```python
from build123d import *

# Parameters (mm, degrees)
SKETCH1_W           = 6.35
SKETCH1_H           = 241.3
BOSS_EXTRUDE1_DEPTH = 71.12
SKETCH2_W           = 6.35
SKETCH2_H           = 22.86
SKETCH2_H_2         = 25.4
CUT_EXTRUDE1_DEPTH  = 6.35
SKETCH3_W           = 6.35
SKETCH3_H           = 50.8
SKETCH3_H_2         = 25.4
CUT_EXTRUDE2_DEPTH  = 6.35
SKETCH4_W           = 19.05
SKETCH4_H           = 19.05
CUT_EXTRUDE3_DEPTH  = 7.35


with BuildPart() as part:
    # Sketch1 → Boss-Extrude1 (new body)
    with BuildSketch(Plane.XY):
        with Locations((-136.525, -120.65)):
            Rectangle(SKETCH1_W, SKETCH1_H)
    extrude(amount=-BOSS_EXTRUDE1_DEPTH)

    # Sketch2 → Cut-Extrude1 (cut)
    with BuildSketch(Plane(origin=(-133.35, 0, 0), x_dir=(0, 0, -1), z_dir=(1, 0, 0))):
        with Locations((67.945, -38.1)):
            Rectangle(SKETCH2_W, SKETCH2_H)
        with Locations((67.945, -87.63)):
            Rectangle(SKETCH2_W, SKETCH2_H_2)
        with Locations((67.945, -138.43)):
            Rectangle(SKETCH2_W, SKETCH2_H_2)
        with Locations((67.945, -201.93)):
            Rectangle(SKETCH2_W, SKETCH2_H_2)
    extrude(amount=-CUT_EXTRUDE1_DEPTH, mode=Mode.SUBTRACT)

    # Sketch3 → Cut-Extrude2 (cut)
    with BuildSketch(Plane(origin=(-133.35, 0, 0), x_dir=(0, 0, -1), z_dir=(1, 0, 0))):
        with Locations((3.175, -190.5)):
            Rectangle(SKETCH3_W, SKETCH3_H)
        with Locations((3.175, -127)):
            Rectangle(SKETCH3_W, SKETCH3_H_2)
        with Locations((3.175, -63.5)):
            Rectangle(SKETCH3_W, SKETCH3_H)
    extrude(amount=-CUT_EXTRUDE2_DEPTH, mode=Mode.SUBTRACT)

    # Sketch4 → Cut-Extrude3 (cut, through all)
    with BuildSketch(Plane.ZY.offset(139.7)):
        with Locations((-48.895, -15.875)):
            Rectangle(SKETCH4_W, SKETCH4_H)
    extrude(amount=-CUT_EXTRUDE3_DEPTH, mode=Mode.SUBTRACT)


solid = part.part
```
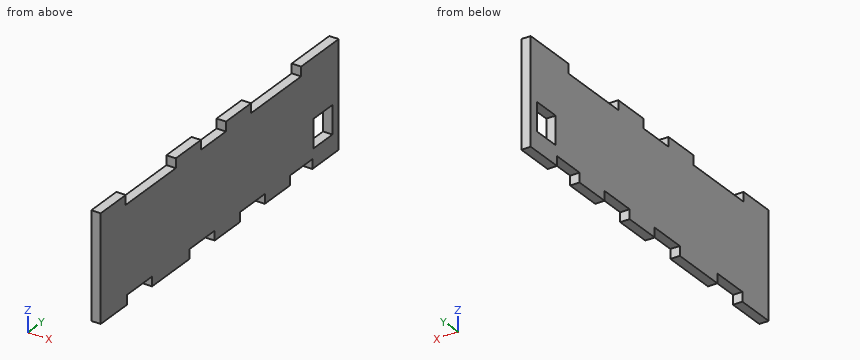
The listing builds one solid part. Answer for the finished solid, in the listing's coordinates (mm). Give positions to 0.01 mm unless a question says otherwise; leave off trailing zeros. Loops run counter-clockwise (first coordinate to the right, second up) from the corner with the lowest first, then second, coordinate; pieces in that order, holes last. Notation, with made-up numbers: (-27.5, -36.75) - (0.5, -36.75) arc R21 cw to (0.5, -9.75) - close; hole circle Ø10 at (-38, 52.5). An arc over 180 degrees is marked (long way). Return JSON: item names as keys, results as strings. Group by question number.
1. Find section A-A (z = -54.5). Write down the section's boundary in (x, y).
2. Find section B-B (y = -47). Write down the section's boundary in (x, z), then the cut area to 3 significant figures.
3. Straight lines are drawn through the part: line 1 (Y direction, x = -137.25, z = -65.5); line 2 (Y direction, x = -134.75, z = -4); line 3 (Y direction, x = -138.5, z = -53). For each, find the intervals that lie inside material, in ascending order. Write a range as [from, to].
4. Find section C-C (y = -143.5). Write down the section's boundary in (x, z), then the cut area to 3 significant figures.
5. Given pin 1 Ø1.9 at (x, y) = (-136, -66) entering from +Z, flat-ended and moving along its own axis, determine where the tip first touches the part or whether it passes through.
Verdict:
{
 "1": {"outline": "(-139.7, -241.3) - (-133.35, -241.3) - (-133.35, -25.4) - (-139.7, -25.4) - close; (-139.7, -6.35) - (-133.35, -6.35) - (-133.35, 0) - (-139.7, 0) - close"},
 "2": {"outline": "(-139.7, -64.77) - (-133.35, -64.77) - (-133.35, -6.35) - (-139.7, -6.35) - close", "area": "371 mm^2"},
 "3": {"line 1": "y = [-241.3, -214.63], [-189.23, -151.13], [-125.73, -100.33], [-74.93, -49.53], [-26.67, 0]", "line 2": "y = [-241.3, -215.9], [-165.1, -139.7], [-114.3, -88.9], [-38.1, 0]", "line 3": "y = [-241.3, -25.4], [-6.35, 0]"},
 "4": {"outline": "(-139.7, -64.77) - (-133.35, -64.77) - (-133.35, 0) - (-139.7, 0) - close", "area": "411 mm^2"},
 "5": {"pin 1": "stops at z = -6.35"}
}
